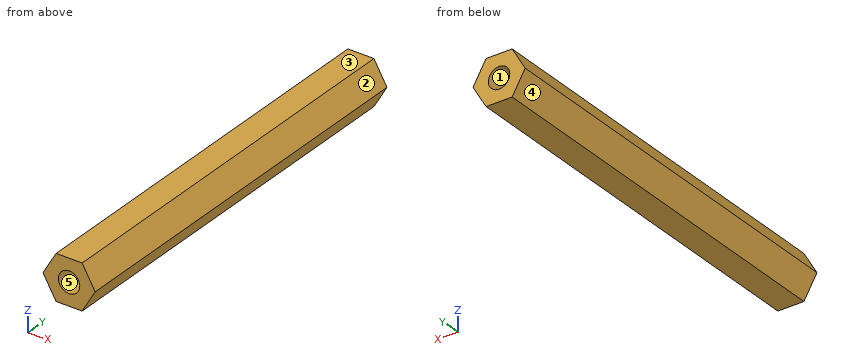
```python
from build123d import *

# Parameters (mm, degrees)
BOSS_EXTRU_1_DEPTH      = 24.5
BOSS_EXTRU_1_DEPTH_BACK = 24.5


with BuildPart() as part:
    # Esquisse1 → Boss.-Extru.1 (new, two sides: drawn at the far end of the back side and taken through both)
    with BuildSketch(Plane(origin=(0, 0, 0), x_dir=(1, 0, 0), z_dir=(0, 1, 0)).offset(-BOSS_EXTRU_1_DEPTH_BACK)):
        Polygon((3.175426481, 0), (1.58771324, 2.75), (-1.58771324, 2.75), (-3.175426481, 0), (-1.58771324, -2.75), (1.58771324, -2.75), align=None)
    extrude(amount=BOSS_EXTRU_1_DEPTH + BOSS_EXTRU_1_DEPTH_BACK)

    # Esquisse3 → Dégagement M31 (revolve, cut)
    with BuildSketch(Plane(origin=(0, 24.5, 0), x_dir=(0, 0, 1), z_dir=(1, 0, 0))):
        Polygon((0, 0), (0, 7.131118805), (1.3, 6.35), (1.3, 0), align=None)
    d_gagement_m31 = revolve(axis=Axis((0, 30.85, 0), (0, -1, 0)), mode=Mode.SUBTRACT)

    # Symétrie1: Dégagement M31 across plane
    add(d_gagement_m31.mirror(Plane.ZX), mode=Mode.SUBTRACT)


solid = part.part
```
The listing builds one solid part. Answer for the finished solid, in the listing's coordinates (mm). Face numbers are marked on the shaded views. A direction names the side the tool comes from. Give positions to 0.01 mm unless a question says otherwise; leave off trailing zeros. Order: outer loops, then holes, each group sorted by start corner. A loop starts at its lowest first (then second) coordinate and runs counter-clockwise, first axis right, second up.
1) Find section B-B on z = -2.15. Write down the section's boundary in (x, y), then the cut area to 3 significant figures.
Reported:
outline: (-1.93, -24.5) - (1.93, -24.5) - (1.93, 24.5) - (-1.93, 24.5) - close
area: 190 mm2
2) Consider line 1 along Z through (x, y) = (0, 20.5); line 2 along X through (y, z) = (-20.5, 0); line 3 along Z through (x, y) = (1.75, 12). Determine where each line is inside the solid, lowest interval first.
Reported:
line 1: z = -2.75 to -1.3, 1.3 to 2.75
line 2: x = -3.18 to -1.3, 1.3 to 3.18
line 3: z = -2.47 to 2.47
3) Determine the mould class of the marked faces 3, 4 and 5 for opening direction Z: pulls with the +Z half, pulls with the -Z half, needs draft (parallel to the pull), parting line crosses it, or undercut.
Reported:
face 3: pulls with the +Z half
face 4: pulls with the -Z half
face 5: undercut
4) Given P1, Ø2, axis at x = 0, z = 0, coming from the +Y side; P2, Ø1.5, axis at y = 3.5, z = -2, coming from the +X side, each flat-ended and moving along its own axis, determine where each tip first touches the part or whether it passes through.
Reported:
P1: stops at y = 17.97
P2: stops at x = 2.45
5) Find section C-C on z = 1.7. Write down the section's boundary in (x, y).
Reported:
outline: (-2.19, -24.5) - (2.19, -24.5) - (2.19, 24.5) - (-2.19, 24.5) - close
6) Find section A-A on y = -15. Write down the section's boundary in (x, z).
Reported:
outline: (-3.18, 0) - (-1.59, -2.75) - (1.59, -2.75) - (3.18, 0) - (1.59, 2.75) - (-1.59, 2.75) - close
7) For the marked faces 1 and 2, determine the directions among +Z, -Z, +X, -X, +Y, -Y from which every point of the face is accessible in a straight line to the end or side of a thin tool.
Reported:
face 1: +Y
face 2: +Z, +X, +Y, -Y
